Geometry check sheet. Reference: the model listing, model coordinates, mm. A direction names the side the tool comes from. Round coordinates to 2 decimals unless told otherwise and drop trailing zeros. Loops run counter-clockwise (first coordinate to the right, second up) from the corner with the lowest first, then second, coordinate; pieces in that order, holes last. Notation, with made-up numbers: M -15,53 L -9,53 A23 ccw -9,79 Z; hole C 84,58 d4. An arc over 180 degrees is marked long. Use one line per item in the form item = value. Start each with the question number.
1. Cross-section at D-D (y = 2). State how many separate pieces and enclosed holes the cut face has, then the cut area to 3 significant figures.
2. Draft check along Z on faces 1 (the flat face through (-35, 4.65, -56)), 2 (the flat face through (-37.66, 2, -36)), 3 (the cylindrical face through (-34.538, 3.252, -113.074)). Enter one of: pulls with the +Z half, pulls with the -Z half, needs draft (parallel to the pull), parting line crosses it, or undercut.
3. Cross-section at C-C (y = 7.25). Record the boundary of the cut face in (x, z) (3 decimals).
4. Set-up check for faces 4 (the cylindrical face through (-35.462, 3.252, -1.326)), 5 (the flat face through (-40.875, 2, -43)), 6 (the cylindrical face through (-32.514, 9.58, -76.5)): record each of +Z, -Z, +X, -X, +Y, -Y from which the full face is reachable in a straight line by a thin tool's end or side.
5. Material ranges on line 1 (Z direction, x = -35, y = 2.3) (3 decimals); line 2 (Z direction, x = -35, y = 2.05) (3 decimals); line 3 (Y direction, x = -15.5, z = -40), recorded low to high.
6. Go/stop test with flat-tipped pins: pin 1 (1.4 mm diameter, centred on x = -38.5, y = 3, fed in from -Z); pin 2 (10 mm diameter, centred on x = -25, z = -24, fed in from +Y); pin 3 (1.6 mm diameter, centred on y = 2, z = -38, fed in from +X). Record where each tip stops, or that it passes through.
Autodesk Inventor part; units mm, degrees
ref_plane "YZ Plane" through (0, 0, 0) normal (1, 0, 0) x (0, 1, 0)
ref_plane "XZ Plane" through (0, 0, 0) normal (0, 1, 0) x (-1, 0, 0)
ref_plane "XY Plane" through (0, 0, 0) normal (0, 0, 1) x (1, 0, 0)
sketch "Sketch1" plane through (0, 0, 0) normal (0, 1, 0) x (-1, 0, 0)
  line L0 (0, 0) -> (70, 0)
  line L1 (70, 0) -> (70, -114.4)
  line L2 (70, -114.4) -> (0, -114.4)
  line L3 (0, -114.4) -> (0, 0)
  dimension "d0" = 70
  dimension "d1" = 114.4
extrude "Extrusion1" add sketch "Sketch1" along normal blind 4.65
sketch "Sketch2" plane through (0, 4.65, 0) normal (0, 1, 0) x (1, 0, 0)
  line L0 (-70, 0) -> (0, 0)
  line L1 (0, 0) -> (-35, 0)
  line L2 (-35, 0) -> (-35, 16)
  circle A0 centre (-35, 16) radius 2.125
  line L3 (0, 0) -> (0, 114.4)
  line L4 (0, 0) -> (0, 114.4)
  line L5 (0, 57.2) -> (13.6816, 57.2)
  circle A1 centre (-35, 98.4) radius 2.125
  dimension "d4" = 35
  dimension "d5" = 16
  dimension "d6" = 90
  dimension "d7" = 4.25
extrude "Extrusion2" cut sketch "Sketch2" against normal blind 10
fillet "Fillet1" radius 4.65 4 edges at (-35, 4.65, -114.4) (0, 4.65, -57.2) (-35, 4.65, 0) (-70, 4.65, -57.2)
fillet "Fillet2" radius 2 4 edges at (-1.3618, 3.2882, -1.3618) (-68.6382, 3.2882, -1.3618) (-68.6382, 3.2882, -113.0382) (-1.3618, 3.2882, -113.0382)
sketch "Sketch3" plane through (0, 4.65, 0) normal (0, 1, 0) x (1, 0, 0)
  line L0 (0, 0) -> (0, 34.4)
  line L1 (0, 2) -> (0, 112.4)
  line L2 (0, 34.4) -> (-70, 34.4)
  line L3 (-70, 112.4) -> (-70, 2)
  line L4 (-35, 34.4) -> (-29.125, 34.4)
  line L5 (-29.125, 34.4) -> (-40.875, 34.4)
  line L6 (-40.875, 34.4) -> (-40.875, 46.4)
  line L7 (-40.875, 46.4) -> (-29.125, 46.4)
  line L8 (-29.125, 46.4) -> (-29.125, 34.4)
  line L9 (-35, 34.4) -> (-32.34, 34.4)
  line L10 (-32.34, 34.4) -> (-32.34, 36.9)
  line L11 (-32.34, 36.9) -> (-31.09, 36.9)
  line L12 (-31.09, 36.9) -> (-31.09, 38.9)
  line L13 (-31.09, 38.9) -> (-28.2521, 38.9)
  line L14 (-35, 34.4) -> (-35, 32.315)
  line L15 (-37.66, 34.4) -> (-37.66, 36.9)
  line L16 (-37.66, 36.9) -> (-38.91, 36.9)
  line L17 (-38.91, 36.9) -> (-38.91, 38.9)
  line L18 (-38.91, 38.9) -> (-41.7479, 38.9)
  point P0 (-40.875, 38.9)
  point P1 (-29.125, 38.9)
  dimension "d12" = 34.4
  dimension "d13" = 70
  dimension "d14" = 5.875
  dimension "d15" = 11.75
  dimension "d16" = 12
  dimension "d17" = 2.66
  dimension "d18" = 2.5
  dimension "d19" = 1.25
  dimension "d20" = 2
extrude "Extrusion3" cut sketch "Sketch3" against normal blind 10 contours L2 L15 L16 L17 L18 L6 L7 L8 L13 L12 L11 L10
sketch "Sketch4" plane through (0, 4.65, 0) normal (0, 1, 0) x (1, 0, 0)
  line L0 (0, 0) -> (0, 114.4)
  line L1 (0, 2) -> (0, 112.4)
  line L2 (0, 114.4) -> (-35, 114.4)
  line L3 (-2, 114.4) -> (-68, 114.4)
  line L4 (-35, 114.4) -> (-35, 80.4)
  circle A0 centre (-35, 80.4) radius 4.625
  dimension "d23" = 114.4
  dimension "d24" = 34
  dimension "d25" = 9.25
extrude "Extrusion4" add sketch "Sketch4" along normal blind 10
thread "Thread1"
sketch "Sketch5" plane through (-35, 14.65, -80.4) normal (0, 1, 0) x (1, 0, 0)
  circle A0 centre (0, 0) radius 0.5
  point P0 (35, -80.4)
  dimension "d30" = 1
extrude "Extrusion5" cut sketch "Sketch5" against normal blind 3
properties part number "ethernet_coax_plug"
Reported:
q1.separate_pieces = 1
q1.enclosed_holes = 3
q1.area = 7,690 mm²
q2.face_1 = needs draft
q2.face_2 = undercut
q2.face_3 = pulls with the -Z half
q3.outline = C -35,-80.4 d9.25
q4.face_4 = +Z, +X, -X, +Y
q4.face_5 = +Y, -Y
q4.face_6 = +Y
q5.line_1 = -113.792 to -100.525, -96.275 to -46.4, -34.4 to -18.125, -13.875 to -0.608
q5.line_2 = -113.924 to -100.525, -96.275 to -46.4, -34.4 to -18.125, -13.875 to -0.476
q5.line_3 = 0 to 4.65
q6.pin_1 = -113.79
q6.pin_2 = 4.65
q6.pin_3 = -0.16
